For this review, take the finished solid that the model builds, in its own axes (mm). Round coordinates to 2 decimals unless told otherwise and drop trailing zeros. Write each loop counter-clockwise with the first axis right and the second up, starting at its lowest first coordinate (ties: lowest second). Pieces come first, ordered by that corner, then holes. Notation, with made-up numbers: (-4.5, 66) - (2.5, 66) arc R18 cw to (2.5, 74) - close; hole circle Ø8 at (43, 36). An arc over 180 degrees is marked (long way). One line per item, written item: value. Start each with the question number.
Q1. For probe 1 along X at (y, z) = (10, 2.3); probe 2 along X at (y, z) = (15, 1.7); probe 3 along Y at (x, z) = (4, 2.55), list the stretches that pass through material, from the lowest coordinate up.
Q2. Add section A-A on x = 156. Write out the cut boundary in (y, z).
Q3. Mouldability with a two-part tool opening along X and no side actions: class faces 1 (the face through (21.419, 31.548, 2.324)), 2 (the face through (81, 40, 2)), 3 (the face through (0, 20, 2)) as +X half, -X half, draft (parallel to the pull), parting line (faces both ways), or undercut.
Q4. Clearance check with a flat-ended pin moving along its axis: pin 1 Ø5 at (x, y) = (4, 25) entering from +Z. State where the tip first meets the part, or that it passes through.
Q5. Add section C-C on z = 1.85. Give the number of separate pieces and of enclosed holes in the cut face, and give its area (3 significant figures).
Q6. Add section B-B on y = 30. Write out the cut boundary in (x, z), and give its area (3 significant figures).
Solid Edge part; units mm, degrees
sketch "Sketch1" plane through (0, 0, 0) normal (0, 0, 1) x (1, 0, 0)
  line L0 (160, 0) -> (160, 40)
  line L1 (160, 40) -> (0, 40)
  line L2 (0, 40) -> (0, 0)
  line L3 (0, 0) -> (160, 0)
extrude "Protrusion1" add sketch "Sketch1" along normal blind 5
hole "Hole_2" at (20, 10, 5) direction (0, 0, -1) diameter 4.2 end up to next start chamfer 1 start chamfer angle 45 end chamfer 0.6 end chamfer angle 45
hole "Hole1" at (140, 10, 5) direction (0, 0, -1) diameter 4.2 end up to next start chamfer 1 start chamfer angle 45 end chamfer 0.6 end chamfer angle 45
hole "Hole2" at (140, 30, 5) direction (0, 0, -1) diameter 4.2 end up to next start chamfer 1 start chamfer angle 45 end chamfer 0.6 end chamfer angle 45
hole "Hole3" at (20, 30, 5) direction (0, 0, -1) diameter 4.2 end up to next start chamfer 1 start chamfer angle 45 end chamfer 0.6 end chamfer angle 45
hole "Hole_10" at (156, 25, 0) direction (0, 0, 1) diameter 4.2 end up to next start chamfer 0.6 start chamfer angle 45 end chamfer 0.6 end chamfer angle 45
hole "Hole4" at (4, 25, 0) direction (0, 0, 1) diameter 4.2 end up to next start chamfer 0.6 start chamfer angle 45 end chamfer 0.6 end chamfer angle 45
hole "Hole5" at (4, 15, 0) direction (0, 0, 1) diameter 4.2 end up to next start chamfer 0.6 start chamfer angle 45 end chamfer 0.6 end chamfer angle 45
hole "Hole6" at (156, 15, 0) direction (0, 0, 1) diameter 4.2 end up to next start chamfer 0.6 start chamfer angle 45 end chamfer 0.6 end chamfer angle 45
Result set:
1. probe 1: x = 0 to 17.9, 22.1 to 137.9, 142.1 to 160
1. probe 2: x = 0 to 1.9, 6.1 to 153.9, 158.1 to 160
1. probe 3: y = 0 to 12.9, 17.1 to 22.9, 27.1 to 40
2. outline: (0, 0) - (12.3, 0) - (12.9, 0.6) - (12.9, 4.4) - (12.3, 5) - (0, 5) - close; (17.1, 0.6) - (17.7, 0) - (22.3, 0) - (22.9, 0.6) - (22.9, 4.4) - (22.3, 5) - (17.7, 5) - (17.1, 4.4) - close; (27.1, 0.6) - (27.7, 0) - (40, 0) - (40, 5) - (27.7, 5) - (27.1, 4.4) - close
3. face 1: undercut
3. face 2: draft
3. face 3: -X half
4. pin 1: stops at z = 4.8
5. separate pieces: 1
5. enclosed holes: 8
5. area: 6,290 mm^2
6. outline: (0, 0) - (17.3, 0) - (17.9, 0.6) - (17.9, 4) - (16.9, 5) - (0, 5) - close; (22.1, 0.6) - (22.7, 0) - (137.3, 0) - (137.9, 0.6) - (137.9, 4) - (136.9, 5) - (23.1, 5) - (22.1, 4) - close; (142.1, 0.6) - (142.7, 0) - (160, 0) - (160, 5) - (143.1, 5) - (142.1, 4) - close
6. area: 755 mm^2
